```python
from build123d import *

# Parameters (mm, degrees)
F0_R          = 25
F1_DEPTH      = 140
F2_W          = 80
F2_H          = 60
F3_DEPTH      = 30
F3_DEPTH_BACK = 30
F4_W          = 15
F4_H          = 20
F5_DEPTH      = 350
F6_W          = 15
F6_H          = 60
F7_DEPTH      = 50
F8_R          = 20
F9_DEPTH      = 110.001


with BuildPart() as f1:
    # F0 (on Right) → F1 (new body)
    with BuildSketch(Plane.YZ):
        Circle(F0_R)
    extrude(amount=F1_DEPTH)

    # F2 (on Front) → F3 (join, two sides)
    with BuildSketch(Plane.XZ) as f3_sk:
        with Locations((70, 0)):
            Rectangle(F2_W, F2_H)
    extrude(amount=F3_DEPTH)
    extrude(f3_sk.sketch, amount=-F3_DEPTH_BACK)

    # F4 (on face) → F5 (join)
    with BuildSketch(Plane.XZ.offset(30)):
        with Locations((102.5, 20)):
            Rectangle(F4_W, F4_H)
        with Locations((37.5, 20)):
            Rectangle(F4_W, F4_H)
        with Locations((37.5, -20)):
            Rectangle(F4_W, F4_H)
        with Locations((102.5, -20)):
            Rectangle(F4_W, F4_H)
    extrude(amount=F5_DEPTH)

    # F6 (on face) → F7 (join)
    with BuildSketch(Plane.XY.offset(30)):
        with Locations((102.5, -350)):
            Rectangle(F6_W, F6_H)
        with Locations((37.5, -350)):
            Rectangle(F6_W, F6_H)
    extrude(amount=-F7_DEPTH)

    # F8 (on face) → F9 (cut, through all)
    with BuildSketch(Plane.YZ.offset(110)):
        with Locations((-350, 0)):
            Circle(F8_R)
    extrude(amount=-F9_DEPTH, mode=Mode.SUBTRACT)


solid = f1.part
```
The model under review builds one solid part; all positions refer to its coordinate system, in mm. A direction names the side the tool comes from. Give positions to 0.01 mm unless a question says otherwise; leave off trailing zeros. Order: outer loops, then holes, each group sorted by start corner. A loop starts at its lowest first (then second) coordinate and runs counter-clockwise, first axis right, second up. Notation, with made-up numbers: (-35.5, 41) - (15.5, 41) arc R15 cw to (15.5, 59) - close; hole circle Ø4 at (42.25, 85.25). An arc over 180 degrees is marked (long way). Use CSV: the item, a comma, the result in double quotes. Start each with the question number.
Q1. We need section D-D, the plane y = 0. Write out the cut boundary in (x, z).
Q2. We need section B-B, the plane y = -76. Write out the cut boundary in (x, z).
Q3. Clearance check with flat-ended pins moving along their axes: pin 1 Ø4 at (y, z) = (-176.5, 21.5) entering from +X; pin 2 Ø18 at (x, z) = (74, 6.5) entering from -Y; pin 3 Ø10 at (x, z) = (17, 2) entering from +Y; pin 4 Ø24 at (y, z) = (-350, 0) entering from -X. State where each tip first meets the part, or that it passes through.
Q4. We need section C-C, the plane z = 0. Write out the cut boundary in (x, y).
Q5. Tool access review of faces 4 (the flat face through (45, -203, -14)), 5 (the flat face through (102, -320, 0)), 6 (the cylindrical face through (14.79, 23.846, 7.509)): name each direction out of +Z, -Z, +X, -X, +Y, -Y from which nothing blocks a thin tool from reaching the whole face with its end or side.
Q6. We need section A-A, the plane x = 103. Write out the cut boundary in (y, z), and give its area (3 significant figures).
Q7. The part is to be moulded in two halves that separate along Z. For faces 1 (the cylindrical face through (102.605, -331.525, -7.66)), 2 (the cylindrical face through (124.79, 23.846, 7.509)), 3 (the flat face through (37, -380, 0)), say which applies: +Z half, -Z half, draft (parallel to the pull), parting line (faces both ways), or undercut.
Q8. To check wall thickness, follow line 1 along Z through (x, y) = (102.5, -350); line 2 along X through (y, z) = (-158, 19); line 3 along Z through (x, y) = (34.5, -308). State the ranges of each line that lie inside material, in increasing order. Write a range as [from, to].
Outcome:
1,outline,"(0, -25) - (30, -25) - (30, -30) - (110, -30) - (110, -25) - (140, -25) - (140, 25) - (110, 25) - (110, 30) - (30, 30) - (30, 25) - (0, 25) - close"
2,outline,"(30, -30) - (45, -30) - (45, -10) - (30, -10) - close; (30, 10) - (45, 10) - (45, 30) - (30, 30) - close; (95, -30) - (110, -30) - (110, -10) - (95, -10) - close; (95, 10) - (110, 10) - (110, 30) - (95, 30) - close"
3,pin 1,"stops at x = 110"
3,pin 2,"stops at y = -30"
3,pin 3,"stops at y = 25"
3,pin 4,"passes through"
4,outline,"(0, -25) - (30, -25) - (30, -30) - (110, -30) - (110, -25) - (140, -25) - (140, 25) - (110, 25) - (110, 30) - (30, 30) - (30, 25) - (0, 25) - close; (30, -380) - (45, -380) - (45, -370) - (30, -370) - close; (30, -330) - (45, -330) - (45, -320) - (30, -320) - close; (95, -380) - (110, -380) - (110, -370) - (95, -370) - close; (95, -330) - (110, -330) - (110, -320) - (95, -320) - close"
5,face 4,"+Z, -Z, -Y"
5,face 5,"+X, -X"
5,face 6,"-X"
6,outline,"(-380, -30) - (30, -30) - (30, 30) - (-380, 30) - close; hole circle Ø40 at (-350, 0); hole (-320, -10) - (-30, -10) - (-30, 10) - (-320, 10) - close"
6,area,"17,500 mm^2"
7,face 1,"undercut"
7,face 2,"parting line"
7,face 3,"draft"
8,line 1,"z = [-30, -20], [20, 30]"
8,line 2,"x = [30, 45], [95, 110]"
8,line 3,"z = [-30, -10], [10, 30]"
